The model under review builds one solid part; all positions refer to its coordinate system, in mm. A direction names the side the tool comes from. Round coordinates to 2 decimals unless told otherwise and drop trailing zeros. Loops run counter-clockwise (first coordinate to the right, second up) from the corner with the lowest first, then second, coordinate; pieces in that order, holes last. Notation, with made-up numbers: M 43.5,77 L 47.5,77 A15 ccw 47.5,83 Z; hole C -1,30.25 d8. An arc over 180 degrees is marked long. Use a Markdown table: item, result. Add a question column.
```python
from build123d import *

# Parameters (mm, degrees)
F1_DEPTH = 6
F2_R     = 2.99999
F3_R     = 3
F4_R     = 1.5
F5_R     = 1.5
F6_DEPTH = 25


# Not quite as in the source:
# - a fillet or chamfer is up to 0.001 mm smaller than in the source, because OpenCascade refuses the exact size


with BuildPart() as f1:
    # F0 (on Top) → F1 (new body)
    with BuildSketch(Plane.XY):
        Polygon((15, 1.5), (12.5, 4), (-23, 4), (-23, 1.5), (9, 1.5), (9, -1.5), (-23, -1.5), (-23, -4), (12.5, -4), (15, -1.5), (23, -1.5), (23, 1.5), align=None)
    extrude(amount=F1_DEPTH)

    # F2 (radius 3 in the source; OpenCascade refuses exactly that, so slightly less here)
    f2_edges = [f1.edges().sort_by_distance(p)[0] for p in [
        (-23, -2.75, 6),
        (-23, 2.75, 6),
        (23, 0, 6),
        (23, 0, 0),
        (-23, 2.75, 0),
        (-23, -2.75, 0),
    ]]
    fillet(f2_edges, radius=F2_R)

    # F3
    f3_edges = [f1.edges().sort_by_distance(p)[0] for p in [
        (12.5, 4, 3),
        (15, 1.5, 3),
        (15, -1.5, 3),
        (12.5, -4, 3),
    ]]
    fillet(f3_edges, radius=F3_R)

    # F4 (on face) + F5 (on face) → F6 (cut)
    with BuildSketch(Plane.XZ.offset(4)):
        with Locations((-20, 3)):
            Circle(F4_R)
        with Locations((-13, 3)):
            Circle(F4_R)
        with Locations((-6, 3)):
            Circle(F4_R)
        with Locations((1, 3)):
            Circle(F4_R)
    with BuildSketch(Plane.XZ.offset(1.5)):
        with Locations((20, 3)):
            Circle(F5_R)
    extrude(amount=-F6_DEPTH, mode=Mode.SUBTRACT)


solid = f1.part
```
(1) Consider section B-B, the plane x = -4. Give the boundary of the cut face in (y, z), then the cut area to 3 significant figures.
(2) Draft analysis for pull direction Z (two halves, no side actions). For faces 4 (the face through (-7, -1.5, 1)), 5 (the face through (0.675, -2.768, 1.536)), 6 (the face through (-21.5, -2.77, 3.07)), 7 (the face through (0, 2, 0)), state which applies: released by +Z, released by -Z, zero draft, split by the parting line, or undercut.
(3) Consider section D-D, the plane x = 1.5. Give the boundary of the cut face in (y, z), then the cut area to 3 significant figures.
(4) Insertion check: pin 1 Ø2.5 at (x, z) = (-6, 3) entering from -Y; pin 2 Ø1.8 at (x, z) = (19, 3) entering from -Y; pin 3 Ø1.8 at (x, z) = (19, 2.5) entering from +Y; pin 4 Ø2 at (y, z) = (-2, 2) entering from +X. Each pin has a flat end and moves straight along its axis. Give the tip position at first contact, or say it passes through.
(5) Consider section C-C, the plane z = 0.7. Give the boundary of the cut face in (x, y).
(6) For faces 1 (the face through (22.14, 0.02, 5.1)), 2 (the face through (18, -1.5, 3)), 3 (the face through (18, 1.5, 3)), list the 3-axis set-ups (+Z, -Z, +X, -X, +Y, -Y) from which the entire face can be reached by the end or side of a thin tool; tool diameter is ignored.
(7) Consider section A-A, the plane x = -13. Give the boundary of the cut face in (y, z), then the cut area to 3 significant figures.
(8) To check wall thickness, follow probe 1 along Z at (x, y) = (1, 3.5); probe 2 along Y at (x, z) = (5.5, 4); probe 3 along X at (y, z) = (-3.25, 3.2). State the ranges of each line that lie inside material, in increasing order.
Found:
| question | item | result |
|---|---|---|
| 1 | outline | M -4,0 L -1.5,0 L -1.5,6 L -4,6 Z; M 1.5,0 L 4,0 L 4,6 L 1.5,6 Z |
| 1 | area | 30.0 mm^2 |
| 2 | face 4 | zero draft |
| 2 | face 5 | undercut |
| 2 | face 6 | undercut |
| 2 | face 7 | released by -Z |
| 3 | outline | M -4,0 L -1.5,0 L -1.5,1.59 L -4,1.59 Z; M -4,4.41 L -1.5,4.41 L -1.5,6 L -4,6 Z; M 1.5,0 L 4,0 L 4,1.59 L 1.5,1.59 Z; M 1.5,4.41 L 4,4.41 L 4,6 L 1.5,6 Z |
| 3 | area | 15.9 mm^2 |
| 4 | pin 1 | passes through |
| 4 | pin 2 | stops at y = -1.5 |
| 4 | pin 3 | stops at y = 1.5 |
| 4 | pin 4 | stops at x = 23 |
| 5 | outline | M -21.93,-4 L 11.26,-4 A3 ccw 13.38,-3.12 L 14.12,-2.38 A3 cw 16.24,-1.5 L 21.93,-1.5 L 21.93,1.5 L 16.24,1.5 A3 cw 14.12,2.38 L 13.38,3.12 A3 ccw 11.26,4 L -21.93,4 L -21.93,1.5 L 9,1.5 L 9,-1.5 L -21.93,-1.5 Z |
| 6 | face 1 | +Z, +X, +Y, -Y |
| 6 | face 2 | +Z, -Z, +X, -Y |
| 6 | face 3 | +Z, -Z, +X, +Y |
| 7 | outline | M -4,0 L -1.5,0 L -1.5,1.5 L -4,1.5 Z; M -4,4.5 L -1.5,4.5 L -1.5,6 L -4,6 Z; M 1.5,0 L 4,0 L 4,1.5 L 1.5,1.5 Z; M 1.5,4.5 L 4,4.5 L 4,6 L 1.5,6 Z |
| 7 | area | 15.0 mm^2 |
| 8 | probe 1 | z = 0 to 1.5, 4.5 to 6 |
| 8 | probe 2 | y = -4 to -1.5, 1.5 to 4 |
| 8 | probe 3 | x = -22.99 to -21.49, -18.51 to -14.49, -11.51 to -7.49, -4.51 to -0.49, 2.49 to 13.24 |
